Autodesk Inventor part; units mm, degrees
ref_plane "YZ Plane" through (0, 0, 0) normal (1, 0, 0) x (0, 1, 0)
ref_plane "XZ Plane" through (0, 0, 0) normal (0, 1, 0) x (-1, 0, 0)
ref_plane "XY Plane" through (0, 0, 0) normal (0, 0, 1) x (1, 0, 0)
sketch "Sketch1" plane through (0, 0, 0) normal (0, 0, 1) x (1, 0, 0)
  line L0 (-85, -102.5) -> (85, -102.5)
  line L1 (85, -102.5) -> (85, 102.5)
  line L2 (85, 102.5) -> (-85, 102.5)
  line L3 (-85, 102.5) -> (-85, -102.5)
  line L4 (-85, -102.5) -> (85, 102.5) construction
  line L5 (85, -102.5) -> (-85, 102.5) construction
  circle A0 centre (0, -32.5) radius 42.5
  point P0 (0, 0)
  point P1 (0, -102.5)
  dimension "d0" = 170
  dimension "d1" = 205
  dimension "d22" = 85
  dimension "d61" = 70
extrude "Plate1" add sketch "Sketch1" along normal blind 3
sketch "Sketch5" plane through (82, 102.5, 0) normal (1, 0, 0) x (0, 1, 0)
  line L0 (-205, 0) -> (0, 0)
  line L1 (0, 0) -> (0, 167)
  line L2 (0, 167) -> (-205, 167)
  line L3 (-205, 167) -> (-205, 0)
edge flange "Flange2" height 167 angle 90 thickness 3 bend radius 5 thickness toward (1, 0, 0) relief round relief width 3 relief depth 1.5 edges at (85, 0, 3) wall of the first edge with corners at (82, -102.5, 0) (82, 102.5, 0) (82, 102.5, 167) (82, -102.5, 167)
bend "Bend2"
corner "Corner2"
sketch "Sketch6" plane through (85, -102.5, 167) normal (1, 0, 0) x (0, 0, -1)
  line L0 (159, 0) -> (159, 205)
  line L1 (0, 205) -> (159, 205)
  line L2 (0, 0) -> (0, 205)
  line L3 (159, 0) -> (0, 0)
  circle A0 centre (79.5, 95) radius 42.5
  point P0 (167, 102.5)
  point P1 (79.5, 205)
  dimension "d33" = 85
  dimension "d60" = 95
extrude "Cut1" cut sketch "Sketch6" against normal blind 3 contours A0
sketch "Sketch7" plane through (85, -102.5, 167) normal (1, 0, 0) x (0, 0, -1)
  circle A0 centre (47, 151.2917) radius 6.5
  circle A1 centre (79.5, 95) radius 42.5
  circle A2 centre (79.5, 95) radius 65 construction
  line L0 (79.5, 95) -> (79.5, 137.5)
  line L1 (79.5, 95) -> (47, 151.2917)
  point P0 (167, 102.5)
  dimension "d37" = 130
  dimension "d36" = 13
  dimension "d81" = 30
extrude "Cut2" cut sketch "Sketch7" against normal blind 3 contours A0
pattern_circular "Circular Pattern1" count 6 over 360 about axis through (85, -7.5, 87.5) along (-1, 0, 0) of "Cut2"
sketch "Sketch8" plane through (0, 0, 3) normal (0, 0, 1) x (1, 0, 0)
  circle A0 centre (-32.5, 23.7917) radius 6.5
  circle A1 centre (0, -32.5) radius 65 construction
  circle A2 centre (0, -32.5) radius 42.5
  line L0 (0, 10) -> (0, -32.5)
  line L1 (0, -32.5) -> (-32.5, 23.7917)
  dimension "d44" = 130
  dimension "d43" = 13
  dimension "d82" = 30
extrude "Cut3" cut sketch "Sketch8" against normal blind 3 contours A0
pattern_circular "Circular Pattern2" count 6 over 360 about axis through (0, -32.5, 0) along (0, 0, 1) of "Cut3"
sketch "Sketch10" plane through (85, -102.5, 167) normal (1, 0, 0) x (0, 0, -1)
  circle A0 centre (41.5, 196) radius 6.5
  circle A1 centre (121.5, 196) radius 6.5
  line L0 (159, 205) -> (0, 205)
  line L1 (81.5, 200.962) -> (81.5, 182.1235)
  point P0 (167, 102.5)
  dimension "d62" = 13
  dimension "d63" = 9
  dimension "d64" = 80
  dimension "d72" = 81.5
extrude "Cut4" cut sketch "Sketch10" against normal blind 3
sketch "Sketch11" plane through (0, 0, 3) normal (0, 0, 1) x (1, 0, 0)
  circle A0 centre (-40, 93.5) radius 6.5
  circle A1 centre (40, 93.5) radius 6.5
  line L0 (0, 102.5) -> (0, 73.9677)
  line L1 (-85, 102.5) -> (77, 102.5)
  point P0 (0, 0)
  dimension "d67" = 13
  dimension "d68" = 80
  dimension "d69" = 9
extrude "Cut5" cut sketch "Sketch11" against normal blind 3
equation "\"d33\" = d22"
equation "\"d34\" = Thickness"
equation "\"d38\" = Thickness"
equation "\"d45\" = Thickness"
equation "\"d65\" = Thickness"
equation "\"d70\" = Thickness"
equation "\"d2\" = Thickness"
equation "\"d23\" = BendReliefWidth"
equation "\"d24\" = BendReliefDepth"
equation "\"d25\" = MinimumRemnant"
equation "\"d26\" = TransitionRadius"
equation "\"d29\" = BendRadius"
equation "\"d30\" = CornerReliefSize"
equation "\"d31\" = GapSize"
equation "\"d32\" = JacobiRadiusSize"
equation "\"BendReliefWidth\" = Thickness"
equation "\"BendReliefDepth\" = 0.5 * Thickness"
equation "\"CornerReliefSize\" = 4 * Thickness"
equation "\"MinimumRemnant\" = 2 * Thickness"
equation "\"TransitionRadius\" = BendRadius"
equation "\"JacobiRadiusSize\" = BendRadius"
equation "\"GapSize\" = Thickness"
properties part number "drain wall with flange" material "Stainless Steel"
Source: CAD feature listing. Evaluate the final solid. Frame: model axes, mm. A direction names the side the tool comes from. Give positions to 0.01 mm unless a question says otherwise; leave off trailing zeros. Write each loop counter-clockwise with the first axis right and the second up, starting at its lowest first coordinate (ties: lowest second). Pieces come first, ordered by that corner, then holes. Notation, with made-up numbers: (0, -21.5) -> (29, -21.5) arc R17 cw to (29, -10.5) -> close; hole circle Ø5 at (88, 42.25). An arc over 180 degrees is marked (long way). Return JSON: item names as keys, results as strings. Group by question number.
1. Access query for faces 4 (the face through (-5, 24, 3)), 5 (the face through (-63.591, -26.155, 1.521)). Directions: +Z, -Z, +X, -X, +Y, -Y. A direction counts if a zero-diameter tool reaches every point of the face in a straight line with its end or side. Return the directions, or none.
2. Pin query (flat end, axial travel): pin 1 Ø21 at (x, y) = (65, -32.5) entering from +Z; pin 2 Ø8 at (x, y) = (-40, 93.5) entering from +Z (1 decimal); pin 3 Ø17 at (y, z) = (93.5, 125.5) entering from -X. Return the tip coordinate at first contact, or that it passes through.
3. Section C-C, the plane z = 87.5. Output: boundary loops of the cut face in (x, y), then the cut area to 3 significant figures.
4. Mould query, pull axis X, two halves, no side actions, for faces 1 (the face through (82, 24, 122)), 2 (the face through (-9.21, 8.99, 1.48)), 3 (the face through (83.52, -23.78, 48.24)). Classes: +X half, -X half, draft (parallel to the pull), parting line (faces both ways), or undercut.
5. Section B-B, the plane x = 0. Output: boundary loops of the cut face in (y, z), then the cut area to 3 significant figures.
6. Section D-D, the plane x = -29.5. Output: boundary loops of the cut face in (y, z), then the cut area to 3 significant figures.
7. Section A-A, the plane y = 93.5. Output: boundary loops of the cut face in (x, z), then the cut area to 3 significant figures.
8. Material intervals for line 1 (Y direction, x = 82.95, z = 87.5); line 2 (Z direction, x = 46.5, y = -54); line 3 (X direction, y = -46, z = 29.5), sorted ascending. Write a range as from..to.
Determined:
{
 "1": {"face 4": "+Z, -X, +Y, -Y", "face 5": "+Z, -Z"},
 "2": {"pin 1": "stops at z = 3", "pin 2": "passes through", "pin 3": "stops at x = 82"},
 "3": {"outline": "(82, -102.5) -> (85, -102.5) -> (85, -50) -> (82, -50) -> close; (82, 35) -> (85, 35) -> (85, 102.5) -> (82, 102.5) -> close", "area": "360 mm2"},
 "4": {"face 1": "-X half", "face 2": "undercut", "face 3": "draft"},
 "5": {"outline": "(-102.5, 0) -> (-75, 0) -> (-75, 3) -> (-102.5, 3) -> close; (10, 0) -> (102.5, 0) -> (102.5, 3) -> (10, 3) -> close", "area": "360 mm2"},
 "6": {"outline": "(-102.5, 0) -> (-94.56, 0) -> (-94.56, 3) -> (-102.5, 3) -> close; (-83.03, 0) -> (-63.09, 0) -> (-63.09, 3) -> (-83.03, 3) -> close; (-1.91, 0) -> (18.03, 0) -> (18.03, 3) -> (-1.91, 3) -> close; (29.56, 0) -> (102.5, 0) -> (102.5, 3) -> (29.56, 3) -> close", "area": "362 mm2"},
 "7": {"outline": "(-85, 0) -> (-46.5, 0) -> (-46.5, 3) -> (-85, 3) -> close; (-33.5, 0) -> (33.5, 0) -> (33.5, 3) -> (-33.5, 3) -> close; (46.5, 0) -> (77, 0) arc R8 ccw to (85, 8) -> (85, 39) -> (82, 39) -> (82, 8) arc R5 cw to (77, 3) -> (46.5, 3) -> close; (82, 52) -> (85, 52) -> (85, 119) -> (82, 119) -> close; (82, 132) -> (85, 132) -> (85, 167) -> (82, 167) -> close", "area": "838 mm2"},
 "8": {"line 1": "y = -102.5..-50, 35..102.5", "line 2": "z = 0..3", "line 3": "x = 82..85"}
}
